Design review of the part built by this model. Coordinates are the model's own, in mm. A direction names the side the tool comes from. Coordinates: 2 decimals unless noted, no trailing zeros. Order: outer loops, then holes, each group sorted by start corner. A loop starts at its lowest first (then second) coordinate and runs counter-clockwise, first axis right, second up. Notation, with made-up numbers: (-34, 29) -> (10, 29) arc R24 cw to (10, 58) -> close; hole circle Ø7 at (-31.5, -13.75). An arc over 180 degrees is marked (long way). Write item = value, one per line.
```python
from build123d import *

# Parameters (mm, degrees)
SKETCH1_R           = 50
BOSS_EXTRUDE1_DEPTH = 78.5
BOSS_EXTRUDE2_DEPTH = 8
LPATTERN1_COUNT     = 2
LPATTERN1_PITCH     = 36.66
BOSS_EXTRUDE3_DEPTH = 8
LPATTERN2_COUNT     = 2
LPATTERN2_PITCH     = 36.66


with BuildPart() as part:
    # Sketch1 → Boss-Extrude1 (new body)
    with BuildSketch(Plane(origin=(0, 0, 0), x_dir=(1, 0, 0), z_dir=(0, 1, 0))):
        Circle(SKETCH1_R)
    extrude(amount=BOSS_EXTRUDE1_DEPTH)

    # Sketch2 → Boss-Extrude2 (add, symmetric)
    with BuildSketch(Plane.XY.offset(9.165)):
        with BuildLine():
            Line((0, 78.5), (-24.07, 78.5))
            Line((-24.07, 78.5), (-24.07, 81))
            ThreePointArc((-24.07, 81), (-29.743402859, 89.87202212), (-19.309747906, 91.3))
            Line((-19.309747906, 91.3), (0, 91.3))
            Line((0, 91.3), (0, 78.5))
        make_face()
    boss_extrude2 = extrude(amount=BOSS_EXTRUDE2_DEPTH, both=True)

    # LPattern1: Boss-Extrude2 ×2
    with Locations(*[(0, 0, -i * LPATTERN1_PITCH) for i in range(1, LPATTERN1_COUNT)]):
        add(boss_extrude2)

    # Sketch3 → Boss-Extrude3 (add, symmetric)
    with BuildSketch(Plane.XY.offset(27.495)):
        with BuildLine():
            Line((0, 91.3), (15.309747906, 91.3))
            ThreePointArc((15.309747906, 91.3), (25.743402859, 89.87202212), (20.07, 81))
            Line((20.07, 81), (20.07, 78.5))
            Line((20.07, 78.5), (0, 78.5))
            Line((0, 78.5), (0, 91.3))
        make_face()
    boss_extrude3 = extrude(amount=BOSS_EXTRUDE3_DEPTH, both=True)

    # LPattern2: Boss-Extrude3 ×2
    with Locations(*[(0, 0, -i * LPATTERN2_PITCH) for i in range(1, LPATTERN2_COUNT)]):
        add(boss_extrude3)


solid = part.part
```
(1) We need section A-A (y = 87.25). Write out the cut boundary in (x, z) (3 decimals), and give its area (3 significant figures).
Report:
outline = (-30.32, -35.495) -> (0, -35.495) -> (0, -19.495) -> (-30.32, -19.495) -> close; (-30.32, 1.165) -> (0, 1.165) -> (0, 17.165) -> (-30.32, 17.165) -> close; (0, -17.165) -> (26.32, -17.165) -> (26.32, -1.165) -> (0, -1.165) -> close; (0, 19.495) -> (26.32, 19.495) -> (26.32, 35.495) -> (0, 35.495) -> close
area = 1,810 mm²
(2) For L1, parallel to Z at x = -29, y = 85.5 (3 decimals); L2, parallel to Y at x = -14.5, z = -36.5; L3, parallel to Z at x = 15.5, y = 85 (3 decimals), list the stretches that pass through material, from the lowest coordinate up.
Report:
L1 = -35.495 to -19.495, 1.165 to 17.165
L2 = 0 to 78.5
L3 = -17.165 to -1.165, 19.495 to 35.495
(3) We need section D-D (z = -37). Write out the cut boundary in (x, y).
Report:
outline = (-33.63, 0) -> (33.63, 0) -> (33.63, 78.5) -> (-33.63, 78.5) -> close
(4) The part is to be moulded in two halves that separate along Y. For faces 4 (the cylindrical face through (-29.815, 89.712, -27.383)), 5 (the cylindrical face through (25.668, 90.03, 27.607)), 6 (the flat face through (8, 91.3, 28)), 7 (the flat face through (13, 86, -1.165)), say which applies: released by +Y, released by -Y, zero draft, split by the parting line, or undercut.
Report:
face_4 = undercut
face_5 = undercut
face_6 = released by +Y
face_7 = zero draft
(5) For faces 1 (the flat face through (0, 85, 28)), 2 (the flat face through (-10, 91.3, -27)), 3 (the flat face through (13, 86, 35.495)), list the 3-axis set-ups (+Z, -Z, +X, -X, +Y, -Y) from which the entire face can be reached by the end or side of a thin tool; tool diameter is ignored.
Report:
face_1 = +Z, -X, +Y
face_2 = +Z, -Z, +X, +Y
face_3 = +Z, +X, -X, +Y
(6) We need section B-B (x = 22). Write out the cut boundary in (y, z) (3 decimals).
Report:
outline = (0, -44.9) -> (78.5, -44.9) -> (78.5, 44.9) -> (0, 44.9) -> close; (81.305, -17.165) -> (93.195, -17.165) -> (93.195, -1.165) -> (81.305, -1.165) -> close; (81.305, 19.495) -> (93.195, 19.495) -> (93.195, 35.495) -> (81.305, 35.495) -> close
(7) We need section C-C (x = -10.5). Write out the cut boundary in (y, z) (3 decimals), and give its area (3 significant figures).
Report:
outline = (0, -48.885) -> (78.5, -48.885) -> (78.5, -35.495) -> (91.3, -35.495) -> (91.3, -19.495) -> (78.5, -19.495) -> (78.5, 1.165) -> (91.3, 1.165) -> (91.3, 17.165) -> (78.5, 17.165) -> (78.5, 48.885) -> (0, 48.885) -> close
area = 8,080 mm²
(8) Insertion check: pin 1 (2 mm diameter, centred on x = -3.5, y = 76, fed in from +Z); pin 2 (7.5 mm diameter, centred on x = 8.5, z = -12.5, fed in from +Y); pin 3 (4.5 mm diameter, centred on x = 8, y = 82.5, fed in from +Z) (3 decimals); pin 4 (8 mm diameter, centred on x = 9.5, z = -15, fed in from -Y). Each pin has a flat end and moves straight along its axis. Give the tip position at first contact, or say it passes through.
Report:
pin_1 = 49.94
pin_2 = 91.3
pin_3 = 35.495
pin_4 = 0
